```python
from build123d import *

# Parameters (mm, degrees)
SKETCH1_R            = 1.25
BOSS_EXTRUDE1_DEPTH  = 4
FILLET1_R            = 7.5
FILLET1_OF_MIRROR1_R = 7.5


with BuildPart() as part:
    # Sketch1 → Boss-Extrude1 (new body)
    with BuildSketch(Plane.XY):
        with BuildLine():
            Line((-10, -14.45), (7.681, -14.45))
            Line((7.681, -14.45), (7.681, -20.50229958))
            ThreePointArc((7.681, -20.50229958), (21.133001436, -26.074301016), (15.561, -12.62229958))
            Line((15.561, -12.62229958), (10, -12.62229958))
            Line((10, -12.62229958), (10, 0))
            Line((10, 0), (-10, 0))
            Line((-10, 0), (-10, -14.45))
        make_face()
        with Locations((-7.5, -5)):
            Circle(SKETCH1_R, mode=Mode.SUBTRACT)
        with Locations((7.5, -5)):
            Circle(SKETCH1_R, mode=Mode.SUBTRACT)
        with Locations((15.561, -20.50229958)):
            Circle(SKETCH1_R, mode=Mode.SUBTRACT)
    boss_extrude1 = extrude(amount=BOSS_EXTRUDE1_DEPTH)

    # Fillet1
    fillet1_edges = [part.edges().sort_by_distance(p)[0] for p in [
        (7.681, -14.45, 2),
        (10, -12.62229958, 2),
    ]]
    fillet(fillet1_edges, radius=FILLET1_R)

    # Mirror1: Boss-Extrude1 across plane
    add(boss_extrude1.mirror(Plane(origin=(-10, 0, 4), x_dir=(0, 0, 1), z_dir=(0, 1, 0))))

    # Fillet1 of Mirror1
    fillet1_of_mirror1_edges = [part.edges().sort_by_distance(p)[0] for p in [
        (7.681, 14.45, 2),
        (10, 12.62229958, 2),
    ]]
    fillet(fillet1_of_mirror1_edges, radius=FILLET1_OF_MIRROR1_R)


solid = part.part
```
CAD build for the part. Positions are in the model's coordinates, mm. A direction names the side the tool comes from. Round coordinates to 2 decimals unless told otherwise and drop trailing zeros. Order: outer loops, then holes, each group sorted by start corner. A loop starts at its lowest first (then second) coordinate and runs counter-clockwise, first axis right, second up. Notation, with made-up numbers: (88, 21) - (111, 21) arc R29 cw to (111, 42) - close; hole circle Ø3 at (22, -5.75). An arc over 180 degrees is marked (long way). Answer in a Markdown table with one row per item. Add a question column.
(1) Mould opens along X. For faces 1 (the face through (10, 0, 2)), 2 (the face through (6, 0, 0)), 3 (the face through (-8.49, 5.76, 1.97)) say: +X half, -X half, draft (parallel to the pull), parting line (faces both ways), or undercut.
(2) Probe L1, parallel to Y at x = -7.5, z = 2.2; L2, parallel to X at y = 5, z = 1.95; L3, parallel to X at y = 4, z = 1.5. List the from-to ranges inside material, lowest first. Write a range as [from, to].
(3) Band-saw the part on B-B on z = 2.3. Count the separate pieces of the cut face and the enclosed holes in it, and give its area (3 significant figures).
(4) Drop flat-ended pins along their axis: pin 1 Ø2 at (x, y) = (-7.5, 5) entering from +Z; pin 2 Ø1.2 at (y, z) = (-2, 3) entering from +X. Give the stop position or say it passes through.
(5) Band-saw the part on D-D on y = -24. List the corners of the cut face in (x, z), and give its area (3 significant figures).
(6) 3-axis set-ups, long thin cutter, end or side, ignore diameter. For faces 4 (the face through (-5, -14.45, 2)), 5 (the face through (14.6, 21.3, 2)), 6 (the face through (-5, 14.45, 2)): which of +Z, -Z, +X, -X, +Y, -Y reach the whole face in a straight line?
(7) Band-saw the part on A-A on x = -7.5. List the corners of the cut face in (y, z).
Data:
| question | item | result |
|---|---|---|
| 1 | face 1 | +X half |
| 1 | face 2 | draft |
| 1 | face 3 | undercut |
| 2 | L1 | y = [-14.45, -6.25], [-3.75, 3.75], [6.25, 14.45] |
| 2 | L2 | x = [-10, -8.75], [-6.25, 6.25], [8.75, 10] |
| 2 | L3 | x = [-10, -8.25], [-6.75, 6.75], [8.25, 10] |
| 3 | separate pieces | 1 |
| 3 | enclosed holes | 6 |
| 3 | area | 1,000 mm^2 |
| 4 | pin 1 | passes through |
| 4 | pin 2 | stops at x = 10 |
| 5 | outline | (8.5, 0) - (22.62, 0) - (22.62, 4) - (8.5, 4) - close |
| 5 | area | 56.5 mm^2 |
| 6 | face 4 | +Z, -Z, -X, -Y |
| 6 | face 5 | +Z, -Z |
| 6 | face 6 | +Z, -Z, -X, +Y |
| 7 | outline | (-14.45, 0) - (-6.25, 0) - (-6.25, 4) - (-14.45, 4) - close; (-3.75, 0) - (3.75, 0) - (3.75, 4) - (-3.75, 4) - close; (6.25, 0) - (14.45, 0) - (14.45, 4) - (6.25, 4) - close |
